Autodesk Inventor part; units mm, degrees
ref_plane "YZ Plane" through (0, 0, 0) normal (1, 0, 0) x (0, 1, 0)
ref_plane "XZ Plane" through (0, 0, 0) normal (0, 1, 0) x (-1, 0, 0)
ref_plane "XY Plane" through (0, 0, 0) normal (0, 0, 1) x (1, 0, 0)
sketch "Sketch1" plane through (0, 0, 0) normal (0, 1, 0) x (-1, 0, 0)
  line L0 (0, 0) -> (-300, 0)
  line L1 (-300, 0) -> (-300, -23.685)
  line L2 (-300, -23.685) -> (0, -23.685)
  line L3 (0, -23.685) -> (0, 0)
  dimension "d0" = 300
  dimension "d1" = 23.685
extrude "Extrusion1" add sketch "Sketch1" along normal blind 6.5
sketch "Sketch2" plane through (0, 6.5, 0) normal (0, 1, 0) x (1, 0, 0)
  line L0 (0, 23.685) -> (0, 0)
  line L1 (26, 19.3425) -> (32, 19.3425)
  line L2 (33, 18.3425) -> (33, 5.3425)
  line L3 (32, 4.3425) -> (26, 4.3425)
  line L4 (25, 5.3425) -> (25, 18.3425)
  arc A0 (26, 19.3425) -> (25, 18.3425) centre (26, 18.3425) ccw
  arc A1 (25, 5.3425) -> (26, 4.3425) centre (26, 5.3425) ccw
  arc A2 (32, 4.3425) -> (33, 5.3425) centre (32, 5.3425) ccw
  arc A3 (33, 18.3425) -> (32, 19.3425) centre (32, 18.3425) ccw
  point P0 (25, 11.8425)
  point P1 (0, 11.8425)
  dimension "d4" = 1
  dimension "d5" = 15
  dimension "d6" = 8
  dimension "d7" = 25
extrude "Extrusion2" cut sketch "Sketch2" against normal through all
pattern_linear "Rectangular Pattern1" count 5 spacing 14 along (1, 0, 0) of "Extrusion2"
sketch "Sketch3" plane through (0, 0, 0) normal (0, -1, 0) x (1, 0, 0)
  line L0 (0, 0) -> (300, 0)
  line L1 (0, -23.685) -> (0, 0)
  line L2 (300, -23.685) -> (0, -23.685)
  line L3 (16.3, -9.5925) -> (16.3, -14.0925)
  line L4 (0, -14.0925) -> (0, -9.5925)
  line L5 (5, -7.0925) -> (12.3, -7.0925)
  line L6 (12.3, -16.5925) -> (5, -16.5925)
  line L7 (150, 0) -> (150, -23.685) construction
  line L8 (0, -9.5925) -> (5, -9.5925)
  line L9 (12.3, -9.5925) -> (16.3, -9.5925)
  line L10 (16.3, -14.0925) -> (12.3, -14.0925)
  line L11 (5, -14.0925) -> (0, -14.0925)
  line L12 (5, -16.5925) -> (5, -14.0925)
  line L13 (5, -9.5925) -> (5, -7.0925)
  line L14 (12.3, -7.0925) -> (12.3, -9.5925)
  line L15 (12.3, -14.0925) -> (12.3, -16.5925)
  line L16 (283.7, -9.5925) -> (283.7, -14.0925)
  line L17 (300, -14.0925) -> (300, -9.5925)
  line L18 (295, -7.0925) -> (287.7, -7.0925)
  line L19 (287.7, -16.5925) -> (295, -16.5925)
  line L20 (300, -9.5925) -> (295, -9.5925)
  line L21 (287.7, -9.5925) -> (283.7, -9.5925)
  line L22 (283.7, -14.0925) -> (287.7, -14.0925)
  line L23 (295, -14.0925) -> (300, -14.0925)
  line L24 (295, -16.5925) -> (295, -14.0925)
  line L25 (295, -9.5925) -> (295, -7.0925)
  line L26 (287.7, -7.0925) -> (287.7, -9.5925)
  line L27 (287.7, -14.0925) -> (287.7, -16.5925)
  point P0 (16.3, -11.8425)
  point P1 (0, -11.8425)
  point P2 (283.7, -11.8425)
  point P3 (300, -11.8425)
  dimension "d13" = 4.5
  dimension "d14" = 5
  dimension "d15" = 4
  dimension "d16" = 7.3
  dimension "d17" = 2.5
extrude "Extrusion3" cut sketch "Sketch3" against normal through all
sketch "Sketch4" plane through (0, 6.5, 0) normal (0, 1, 0) x (1, 0, 0)
  line L0 (16.3, 14.0925) -> (16.3, 9.5925)
  line L1 (0, 9.5925) -> (0, 0)
  line L2 (89, 18.3425) -> (89, 5.3425)
  circle A0 centre (110, 11.8425) radius 2.25
  circle A1 centre (99, 11.8425) radius 1.5
  point P0 (16.3, 11.8425)
  dimension "d20" = 110
  dimension "d21" = 4.5
  dimension "d22" = 3
  dimension "d23" = 10
extrude "Extrusion4" cut sketch "Sketch4" against normal through all
properties part number "front_pane_middle" material "Plywood, Finish"
Model file for the job. Use its own axes, mm. A direction names the side the tool comes from. Give positions to 0.01 mm unless a question says otherwise; leave off trailing zeros.
1) Tool access for faces 4 (the flat face through (47, 3, -12)), 5 (the flat face through (300, 3, -5)): list every direction of +Z, -Z, +X, -X, +Y, -Y with a clear straight run to the whole face (end or side of a thin tool).
2) Wall check: line 1 (X direction, y = 0.75, z = -17); line 2 (Z direction, x = 99, y = 3) (1 decimal); line 3 (Z direction, x = 110, y = 2.5) (1 decimal). Give the ranges that are in metal, low to high.
3) Flat gauge pins, fed straight in: pin 1 Ø2.5 at (y, z) = (3, -11.5) entering from -X; pin 2 Ø3 at (y, z) = (4.5, -12.5) entering from +X. Where does each tip first touch, or does it go through?
4) Saw through at A-A (y = 5). Count the separate pieces of the cut face and the enclosed holes in it, plus the area to 3 significant figures.
5) Pull direction X, two halves, no side cores. Call faces 1 (the flat face through (0, 3, -19)), 2 (the flat face through (298, 3, -9.592)), 3 (the flat face through (9, 3, -7.092)): +X half, -X half, draft (parallel to the pull), parting line (faces both ways), or undercut.
Answer block:
1. face 4: +Y, -Y
1. face 5: +Z, -Z, +X, +Y, -Y
2. line 1: x = 0 to 25, 33 to 39, 47 to 53, 61 to 67, 75 to 81, 89 to 300
2. line 2: z = -23.7 to -13.3, -10.3 to 0
2. line 3: z = -23.7 to -14.1, -9.6 to 0
3. pin 1: stops at x = 16.3
3. pin 2: stops at x = 283.7
4. separate pieces: 1
4. enclosed holes: 7
4. area: 6,270 mm2
5. face 1: -X half
5. face 2: draft
5. face 3: undercut
